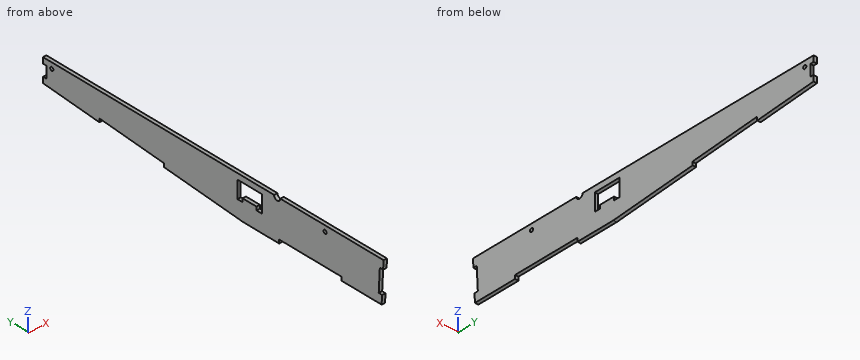
from build123d import *

# Parameters (mm, degrees)
F0_R     = 1.5
F1_DEPTH = 3


with BuildPart() as f1:
    # F0 (on Right) → F1 (new body)
    with BuildSketch(Plane.YZ):
        with BuildLine():
            Line((-144.238283, 7.012537), (-143.843249, -0.525151))
            Line((-143.843249, -0.525151), (-106.134906, -0.525151))
            Line((-106.134906, -0.525151), (-106.134906, 2.574849))
            Line((-106.134906, 2.574849), (-47.581803, 2.574849))
            Line((-47.581803, 2.574849), (-47.581803, -0.525151))
            Line((-47.581803, -0.525151), (-13.843249, -0.525151))
            Line((-13.843249, -0.525151), (60.658704, 5.413919))
            Line((60.658704, 5.413919), (60.420309, 8.404432))
            Line((60.420309, 8.404432), (121.137942, 13.261014))
            Line((121.137942, 13.261014), (121.377632, 10.254247))
            Line((121.377632, 10.254247), (174.322478, 14.474849))
            Line((174.322478, 14.474849), (174.322478, 19.474849))
            Line((174.322478, 19.474849), (171.222478, 19.474849))
            Line((171.222478, 19.474849), (171.222478, 29.474849))
            Line((171.222478, 29.474849), (174.322478, 29.474849))
            Line((174.322478, 29.474849), (174.322478, 34.474849))
            Line((174.322478, 34.474849), (164.322478, 34.474849))
            Line((164.322478, 34.474849), (-42.766357, 34.474849))
            ThreePointArc((-42.766357, 34.474849), (-45.677522, 31.563684), (-48.588687, 34.474849))
            Line((-48.588687, 34.474849), (-85.677522, 34.474849))
            Line((-85.677522, 34.474849), (-145.677522, 34.474849))
            Line((-145.677522, 34.474849), (-145.285002, 26.985128))
            Line((-145.285002, 26.985128), (-142.189251, 27.147369))
            Line((-142.189251, 27.147369), (-141.142531, 7.174779))
            Line((-141.142531, 7.174779), (-144.238283, 7.012537))
        make_face()
        Polygon((-31.22394, 17.474849), (-31.22394, 29.474849), (-8.22394, 29.474849), (-8.22394, 17.474849), (-8.22394, 14.474849), (-13.22394, 14.474849), (-13.22394, 17.474849), (-26.22394, 17.474849), (-26.22394, 14.474849), (-31.22394, 14.474849), align=None, mode=Mode.SUBTRACT)
        with Locations((-90.677522, 29.474849)):
            Circle(F0_R, mode=Mode.SUBTRACT)
        with Locations((166.069406, 29.474849)):
            Circle(F0_R, mode=Mode.SUBTRACT)
    extrude(amount=F1_DEPTH)


solid = f1.part
Geometry check sheet. Reference: the model listing, model coordinates, mm. Give positions to 0.01 mm unless a question says otherwise; leave off trailing zeros. Order: outer loops, then holes, each group sorted by start corner. A loop starts at its lowest first (then second) coordinate and runs counter-clockwise, first axis right, second up. Notation, with made-up numbers: (-10.75, 22.25) - (2.25, 22.25) arc R9 cw to (2.25, 35.25) - close; hole circle Ø6 at (85.5, 13). An arc over 180 degrees is marked (long way). Use one line per item in the form item = value.
1) Depth check by flat-ended pin: pin 1 Ø0.9 at (x, z) = (2, 0.5) entering from -Y; pin 2 Ø1.5 at (x, y) = (1.5, 172.5) entering from -Z; pin 3 Ø1.5 at (x, z) = (2, 25.5) entering from +Y. Enter the tip coordinate at first touch or a pass-through.
Working result:
pin_1 = -143.92
pin_2 = 14.27
pin_3 = 171.22
2) Material ranges on probe 1 along Y at (x, z) = (2.3, 17); probe 2 along Y at (x, z) = (1.6, 29); probe 3 along Y at (x, z) = (1.85, 30), recorded low to high. Write a range as from..to.
Working result:
probe_1 = -141.66..-31.22, -26.22..-13.22, -8.22..174.32
probe_2 = -145.39..-92.1, -89.25..-31.22, -8.22..164.65, 167.49..171.22
probe_3 = -145.44..-92.08, -89.27..164.66, 167.47..174.32
3) Sectioned sample at A-A (x = 1.8). Count the separate pieces of the cut face and the enclosed holes in it, and give its area (3 significant figures).
Working result:
separate_pieces = 1
enclosed_holes = 3
area = 8,970 mm^2
4) Sectioned sample at C-C (y = 115.5). Record the boundary of the cut face in (x, z), and give its area (3 significant figures).
Working result:
outline = (0, 12.81) - (3, 12.81) - (3, 34.47) - (0, 34.47) - close
area = 65.0 mm^2
5) Sectioned sample at B-B (y = -95). Record the boundary of the cut face in (x, z), and give its area (3 significant figures).
Working result:
outline = (0, 2.57) - (3, 2.57) - (3, 34.47) - (0, 34.47) - close
area = 95.7 mm^2
